Can you work these out from the model? Positions are in its coordinate system, mm. A direction names the side the tool comes from. Give positions to 0.01 mm unless a question says otherwise; leave off trailing zeros. Loops run counter-clockwise (first coordinate to the right, second up) from the corner with the lowest first, then second, coordinate; pieces in that order, holes last. Notation, with made-up numbers: M 80.25,2 L 119.25,2 A23 ccw 119.25,10 Z; hole C 7.25,46.5 d2. An arc over 180 degrees is marked long. Answer as a JSON object with one key per item and string values.
```python
from build123d import *

# Parameters (mm, degrees)
BOSS_EXTRUDE1_DEPTH = 2.5
CUT_EXTRUDE1_DEPTH  = 2.5


with BuildPart() as part:
    # Sketch1 one side → Revolve2 (revolve)
    with BuildSketch(Plane.XY):
        with BuildLine():
            ThreePointArc((0, -16.5), (-13.923900316, -8.852965605), (-14.941552797, 7))
            Line((-14.941552797, 7), (-17.663521733, 7))
            ThreePointArc((-17.663521733, 7), (-15.716233646, -10.677078252), (0, -19))
            Line((0, -19), (0, -16.5))
        make_face()
    revolve(axis=Axis((0, -16.5, 0), (0, 1, 0)))

    # Sketch2 → Boss-Extrude1 (add)
    with BuildSketch(Plane(origin=(0, 7, 0), x_dir=(1, 0, 0), z_dir=(0, 1, 0))):
        with BuildLine():
            ThreePointArc((17.663521733, 0), (16.399068955, 6.562814748), (12.786743696, 12.186024194))
            Line((12.786743696, 12.186024194), (12.786743696, 7.729759741))
            ThreePointArc((12.786743696, 7.729759741), (14.392772597, 4.012243385), (14.941552797, 0))
            ThreePointArc((14.941552797, 0), (14.392772597, -4.012243385), (12.786743696, -7.729759741))
            Line((12.786743696, -7.729759741), (12.786743696, -12.186024194))
            ThreePointArc((12.786743696, -12.186024194), (16.399068955, -6.562814748), (17.663521733, 0))
        make_face()
        with BuildLine():
            ThreePointArc((14.941552797, 0), (14.392772597, 4.012243385), (12.786743696, 7.729759741))
            Line((12.786743696, 7.729759741), (12.786743696, -7.729759741))
            ThreePointArc((12.786743696, -7.729759741), (14.392772597, -4.012243385), (14.941552797, 0))
        make_face()
        with BuildLine():
            Line((-12.786743696, 7.729759741), (-12.786743696, 12.186024194))
            ThreePointArc((-12.786743696, 12.186024194), (-17.663521733, 0), (-12.786743696, -12.186024194))
            Line((-12.786743696, -12.186024194), (-12.786743696, -7.729759741))
            ThreePointArc((-12.786743696, -7.729759741), (-14.941552797, 0), (-12.786743696, 7.729759741))
        make_face()
        with BuildLine():
            Line((-12.786743696, -7.729759741), (-12.786743696, 7.729759741))
            ThreePointArc((-12.786743696, 7.729759741), (-14.941552797, 0), (-12.786743696, -7.729759741))
        make_face()
        with BuildLine():
            Line((8.645855328, 12.186024194), (12.786743696, 12.186024194))
            ThreePointArc((12.786743696, 12.186024194), (0, 17.663521733), (-12.786743696, 12.186024194))
            Line((-12.786743696, 12.186024194), (-8.645855328, 12.186024194))
            ThreePointArc((-8.645855328, 12.186024194), (0, 14.941552797), (8.645855328, 12.186024194))
        make_face()
        with BuildLine():
            Line((12.786743696, 7.729759741), (12.786743696, 12.186024194))
            Line((12.786743696, 12.186024194), (8.645855328, 12.186024194))
            ThreePointArc((8.645855328, 12.186024194), (10.9454853, 10.170857955), (12.786743696, 7.729759741))
        make_face()
        with BuildLine():
            Line((-8.645855328, 12.186024194), (-12.786743696, 12.186024194))
            Line((-12.786743696, 12.186024194), (-12.786743696, 7.729759741))
            ThreePointArc((-12.786743696, 7.729759741), (-10.9454853, 10.170857955), (-8.645855328, 12.186024194))
        make_face()
        with BuildLine():
            Line((-12.786743696, -7.729759741), (-12.786743696, -12.186024194))
            Line((-12.786743696, -12.186024194), (-8.645855328, -12.186024194))
            ThreePointArc((-8.645855328, -12.186024194), (-10.9454853, -10.170857955), (-12.786743696, -7.729759741))
        make_face()
        with BuildLine():
            Line((12.786743696, -12.186024194), (12.786743696, -7.729759741))
            ThreePointArc((12.786743696, -7.729759741), (10.9454853, -10.170857955), (8.645855328, -12.186024194))
            Line((8.645855328, -12.186024194), (12.786743696, -12.186024194))
        make_face()
        with BuildLine():
            ThreePointArc((-12.786743696, -12.186024194), (0, -17.663521733), (12.786743696, -12.186024194))
            Line((12.786743696, -12.186024194), (8.645855328, -12.186024194))
            ThreePointArc((8.645855328, -12.186024194), (0, -14.941552797), (-8.645855328, -12.186024194))
            Line((-8.645855328, -12.186024194), (-12.786743696, -12.186024194))
        make_face()
    extrude(amount=BOSS_EXTRUDE1_DEPTH)

    # Sketch3 → Cut-Extrude1 (cut)
    with BuildSketch(Plane(origin=(0, 9.5, 0), x_dir=(1, 0, 0), z_dir=(0, 1, 0))):
        with BuildLine():
            Line((-6.37, 14.38749457), (-6.37, 13.515661286))
            ThreePointArc((-6.37, 13.515661286), (-5.218801949, 14.000503784), (-4.031128874, 14.38749457))
            Line((-4.031128874, 14.38749457), (-6.37, 14.38749457))
        make_face()
        with BuildLine():
            Line((6.37, 14.38749457), (4.031128874, 14.38749457))
            ThreePointArc((4.031128874, 14.38749457), (5.218801949, 14.000503784), (6.37, 13.515661286))
            Line((6.37, 13.515661286), (6.37, 14.38749457))
        make_face()
        with BuildLine():
            ThreePointArc((6.37, -13.515661286), (5.218801949, -14.000503784), (4.031128874, -14.38749457))
            Line((4.031128874, -14.38749457), (6.37, -14.38749457))
            Line((6.37, -14.38749457), (6.37, -13.515661286))
        make_face()
        with BuildLine():
            Line((-6.37, -13.515661286), (-6.37, -14.38749457))
            Line((-6.37, -14.38749457), (-4.031128874, -14.38749457))
            ThreePointArc((-4.031128874, -14.38749457), (-5.218801949, -14.000503784), (-6.37, -13.515661286))
        make_face()
    extrude(amount=-CUT_EXTRUDE1_DEPTH, mode=Mode.SUBTRACT)


solid = part.part
```
1) If we mould it in two halves opening along Z, with no side actions, what happens to faces 1 (the flat face through (13, 9.5, -1)), 2 (the cylindrical face through (-0.06, 8.23, -14.94))? For each: +Z half, -Z half, draft (parallel to the pull), parting line (faces both ways), or undercut.
Answer list:
{"face 1": "draft", "face 2": "undercut"}
2) Will these pins go through, and if not, where does the flat tip stop? pin 1 Ø1 at (y, z) = (9, -14) entering from +X; pin 2 Ø2.5 at (x, z) = (-13.5, 3.5) entering from -Y; pin 3 Ø6 at (x, z) = (-9, -6.5) entering from +Y; pin 4 Ø6 at (x, z) = (-7.5, -10.5) entering from +Y.
Answer list:
{"pin 1": "x = 11.39", "pin 2": "y = -14.14", "pin 3": "y = -8.57", "pin 4": "y = 9.5"}
3) For faces 3 (the flat face through (14, 7, 0)), 4 (the flat face through (-5, 8, -14.387)), which set-ups out of +Z, -Z, +X, -X, +Y, -Y let a thin tool reach every point of the face, with its end or its side?
Answer list:
{"face 3": "none", "face 4": "+Y"}
4) Suppose I cut it at B-B, the plane z = -7. Write out the boundary of the cut face in (x, y).
Answer list:
{"outline": "M -16.22,7 A17.66 ccw long 16.22,7 L 16.22,9.5 L 12.79,9.5 L 12.79,7 L 13.2,7 A14.94 cw long -13.2,7 L -12.79,7 L -12.79,9.5 L -16.22,9.5 Z"}
5) Suppose I cut it at D-D, the plane x = 7.5. Write out the boundary of the cut face in (y, z), and give its area (3 significant figures).
Answer list:
{"outline": "M 7,-15.99 L 9.5,-15.99 L 9.5,-12.92 L 7,-12.92 A14.7 cw long 7,12.92 L 9.5,12.92 L 9.5,15.99 L 7,15.99 A17.46 ccw long Z", "area": "195 mm^2"}
6) Suppose I cut it at C-C, the plane y = -6.25. Write out the boundary of the cut face in (x, z).
Answer list:
{"outline": "C 0,0 d35.89; hole C 0,0 d30.54"}
7) Suppose I cut it at A-A, the plane x = -10.5. Write out the boundary of the cut face in (y, z), and give its area (3 significant figures).
Answer list:
{"outline": "M 7,-14.2 L 9.5,-14.2 L 9.5,-10.63 L 7,-10.63 A12.73 cw long 7,10.63 L 9.5,10.63 L 9.5,14.2 L 7,14.2 A15.84 ccw long Z", "area": "203 mm^2"}
8) Please list where these lines run through material, in increasing order: line 1 along Z through (x, y) = (-4, 5.75); line 2 along X through (y, z) = (-5, 5.5); line 3 along X through (y, z) = (5.5, 4.5). Write a range as from..to.
Answer list:
{"line 1": "-17.66..-14.94, 14.94..17.66", "line 2": "-17.49..-14.73, 14.73..17.49", "line 3": "-17.62..-14.89, 14.89..17.62"}
